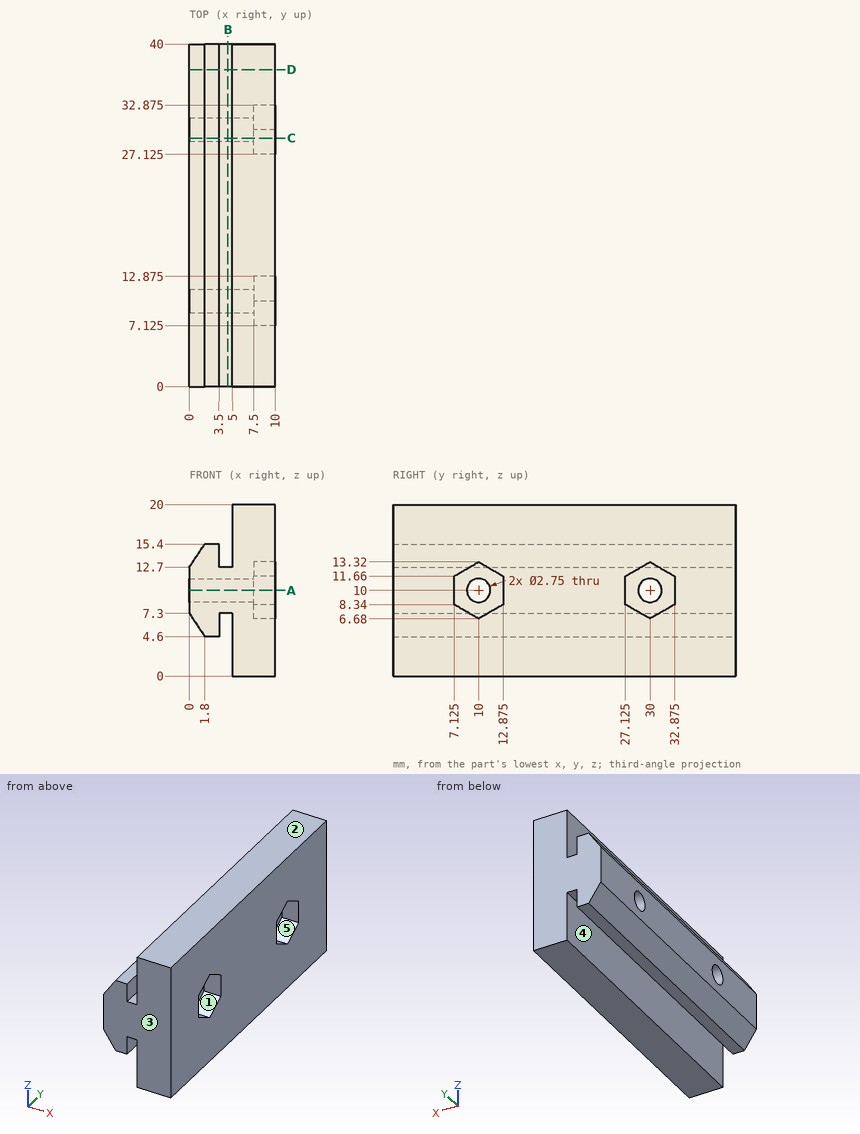
Can you work these out from the drawing? Everything is in mm from the part's minimum corner. A direction names the side the tool comes from. Round coordinates to 2 decimals unless told otherwise and drop trailing zeros. Write each loop counter-clockwise with the first axis right and the second up, starting at its lowest first coordinate (ties: lowest second). Pieces come first, ordered by that corner, then holes. Notation, with made-up numbers: (-15.5, -15) - (28.5, -15) arc R22 cw to (28.5, -7) - close; hole circle Ø6 at (-15, -7.75). An arc over 180 degrees is marked (long way). Write each question's results on one line, items separated by ' | '. Start each with the question number.
1) Suppose I cut it at A-A (z = 10). List the corners of the cut face in (x, y) for me (3 decimals), and give its area (3 significant figures).
2) Suppose I cut it at C-C (y = 29). List the corners of the cut face in (x, z) for me, and give its area (3 significant figures).
3) We'd pull the mould along Y, two halves only. Please class the marked faces 3, 4 and 5: released by +Y, released by -Y, zero draft, split by the parting line, or undercut.
4) Suppose I cut it at D-D (y = 37). List the corners of the cut face in (x, z) for me.
5) Please list where these lines run through material, in increasing order: line 1 (Y direction, x = 2.5, z = 10) (3 decimals); line 2 (Y direction, x = 9.75, z = 10.25) (3 decimals); line 3 (X direction, y = 22.5, z = 1.25).
6) For pin 1 Ø6 at (y, z) = (12.5, 3.5) entering from -X; pin 2 Ø2 at (y, z) = (10, 10) entering from +X; pin 3 Ø2 at (y, z) = (31, 9.5) entering from +X; pin 4 Ø1.2 at (x, y) = (4, 21.5) entering from -Z, each with a flat end and sliding along its axis, tell me the tip position at first contact or that it passes through.
7) Suppose I cut it at B-B (x = 4.5). List the corners of the cut face in (y, z) for me (3 decimals), and give its area (3 significant figures).
8) Which directions (+Z, -Z, +X, -X, +Y, -Y) give clear straight access to the entire face, cutting with the end or side of a thin tool? Please do the marked faces 1 and 2.
Here are the results:
1) outline: (0, 0) - (10, 0) - (10, 7.125) - (7.5, 7.125) - (7.5, 8.625) - (0, 8.625) - close; (0, 11.375) - (7.5, 11.375) - (7.5, 12.875) - (10, 12.875) - (10, 27.125) - (7.5, 27.125) - (7.5, 28.625) - (0, 28.625) - close; (0, 31.375) - (7.5, 31.375) - (7.5, 32.875) - (10, 32.875) - (10, 40) - (0, 40) - close | area: 330 mm2
2) outline: (0, 7.3) - (1.8, 4.6) - (3.5, 4.6) - (3.5, 7.3) - (5, 7.3) - (5, 0) - (10, 0) - (10, 7.26) - (7.5, 7.26) - (7.5, 9.06) - (0, 9.06) - close; (0, 10.94) - (7.5, 10.94) - (7.5, 12.74) - (10, 12.74) - (10, 20) - (5, 20) - (5, 12.7) - (3.5, 12.7) - (3.5, 15.4) - (1.8, 15.4) - (0, 12.7) - close | area: 113 mm2
3) face 3: released by -Y | face 4: zero draft | face 5: undercut
4) outline: (0, 7.3) - (1.8, 4.6) - (3.5, 4.6) - (3.5, 7.3) - (5, 7.3) - (5, 0) - (10, 0) - (10, 20) - (5, 20) - (5, 12.7) - (3.5, 12.7) - (3.5, 15.4) - (1.8, 15.4) - (0, 12.7) - close
5) line 1: y = 0 to 8.625, 11.375 to 28.625, 31.375 to 40 | line 2: y = 0 to 7.125, 12.875 to 27.125, 32.875 to 40 | line 3: x = 5 to 10
6) pin 1: stops at x = 0.53 | pin 2: passes through | pin 3: stops at x = 7.5 | pin 4: stops at z = 4.6
7) outline: (0, 7.3) - (40, 7.3) - (40, 12.7) - (0, 12.7) - close; hole circle Ø2.75 at (10, 10); hole circle Ø2.75 at (30, 10) | area: 204 mm2
8) face 1: +X | face 2: +Z, +X, -X, +Y, -Y
